from build123d import *

# Parameters (mm, degrees)
F0_W     = 37.842602
F0_H     = 26.58715
F1_DEPTH = 12
F2_R     = 8.162544
F3_DEPTH = 25


with BuildPart() as f1:
    # F0 (on Top) → F1 (new body)
    with BuildSketch(Plane.XY):
        Rectangle(F0_W, F0_H)
    extrude(amount=-F1_DEPTH)

    # F2 (on face) → F3 (join)
    with BuildSketch(Plane(origin=(0, 0, -12), x_dir=(1, 0, 0), z_dir=(0, 0, -1))):
        Circle(F2_R)
    extrude(amount=F3_DEPTH)


solid = f1.part
Can you work these out from the model? Positions are in its coordinate system, mm. A direction names the side the tool comes from. Round coordinates to 2 decimals unless told otherwise and drop trailing zeros. Write each loop counter-clockwise with the first axis right and the second up, starting at its lowest first coordinate (ties: lowest second). Pieces come first, ordered by that corner, then holes. Notation, with made-up numbers: M -37,-20 L -9,-20 A34 ccw -9,14 Z; hole C 51,30.5 d11. An arc over 180 degrees is marked long. Use a Markdown table: item, result.
Item 1: Which directions (+Z, -Z, +X, -X, +Y, -Y) give clear straight access to the entire face, cutting with the end or side of a thin tool? Please do faces 1 (the face through (0, -13.294, -6)), 2 (the face through (-9, 0, -12)).
Found:
| item | result |
|---|---|
| face 1 | +Z, -Z, +X, -X, -Y |
| face 2 | -Z |
Item 2: If I drill on line 1 along Z through (x, y) = (-0.5, 8.75); line 2 along Y through (x, z) = (2, -20); line 3 along Y through (x, z) = (-4, -15), over which ranges is the centre line in solid material (lowest first)? Write a range as [from, to].
Found:
| item | result |
|---|---|
| line 1 | z = [-12, 0] |
| line 2 | y = [-7.91, 7.91] |
| line 3 | y = [-7.12, 7.12] |
Item 3: I want a section at D-D (x = -14). List the corners of the cut face in (y, z) for me, and give its area (3 significant figures).
Found:
| item | result |
|---|---|
| outline | M -13.29,-12 L 13.29,-12 L 13.29,0 L -13.29,0 Z |
| area | 319 mm2 |
Item 4: I want a section at B-B (y = 0). List the corners of the cut face in (x, z) for me.
Found:
| item | result |
|---|---|
| outline | M -18.92,-12 L -8.16,-12 L -8.16,-37 L 8.16,-37 L 8.16,-12 L 18.92,-12 L 18.92,0 L -18.92,0 Z |
Item 5: For pin 1 Ø12 at (x, y) = (14.5, -7.5) entering from -Z; pin 2 Ø2 at (y, z) = (-5, -30) entering from -X; pin 3 Ø5 at (y, z) = (-1.5, -18) entering from +X, each with a flat end and sliding along its axis, tell me the tip position at first contact or that it passes through.
Found:
| item | result |
|---|---|
| pin 1 | stops at z = -12 |
| pin 2 | stops at x = -7.12 |
| pin 3 | stops at x = 8.16 |
Item 6: I want a section at C-C (z = -24). List the corners of the cut face in (x, y) for me, and give its area (3 significant figures).
Found:
| item | result |
|---|---|
| outline | C 0,0 d16.33 |
| area | 209 mm2 |
Item 7: I want a section at A-A (x = 0). List the corners of the cut face in (y, z) for me, and give its area (3 significant figures).
Found:
| item | result |
|---|---|
| outline | M -13.29,-12 L -8.16,-12 L -8.16,-37 L 8.16,-37 L 8.16,-12 L 13.29,-12 L 13.29,0 L -13.29,0 Z |
| area | 727 mm2 |
